Verification items for this drawing (mm, ordinates from the low corner). A direction names the side the tool comes from. Give positions to 0.01 mm unless a question says otherwise; leave off trailing zeros. Loops run counter-clockwise (first coordinate to the right, second up) from the corner with the lowest first, then second, coordinate; pieces in that order, holes last. Notation, with made-up numbers: (69, -3.75) -> (124, -3.75) arc R19 ccw to (124, 4.25) -> close; hole circle Ø7 at (-36.75, -29.5). An arc over 180 degrees is marked (long way). Answer as a JSON object with one key per item and string values.
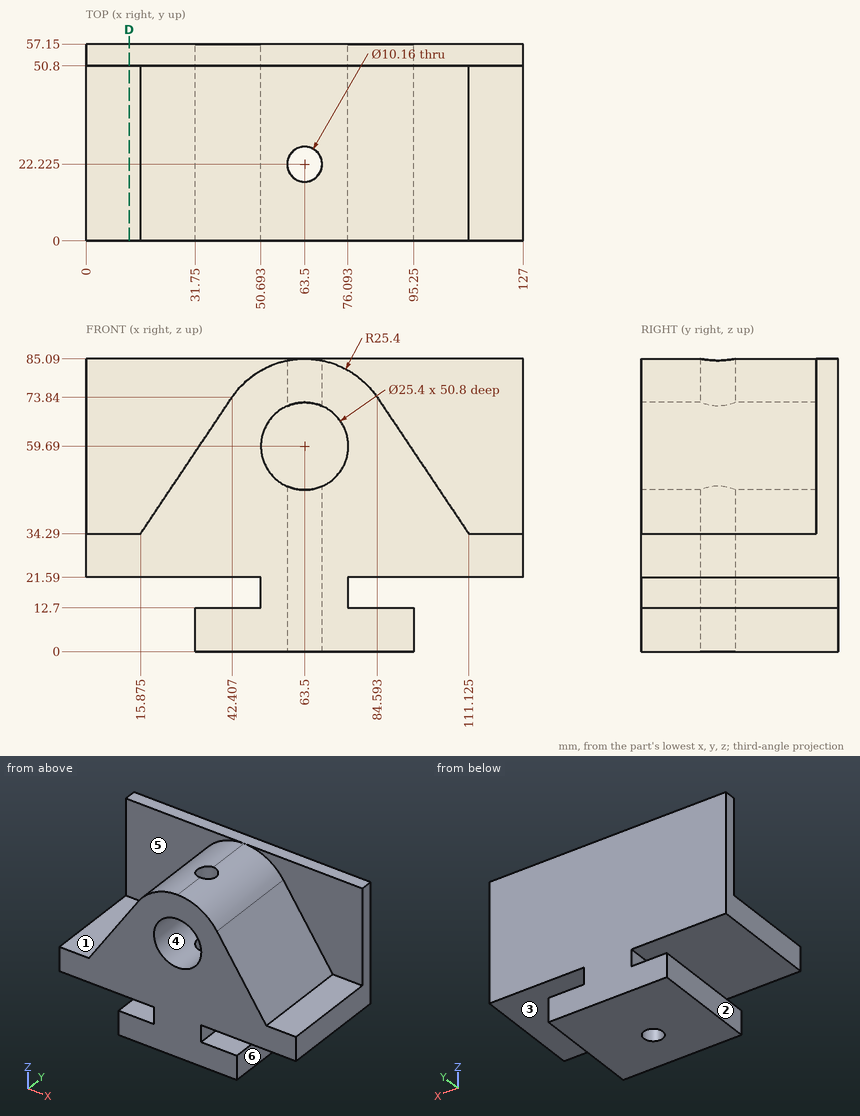
1) Depth check by flat-ended pin: P1, Ø2.5, axis at y = 32, z = 19, coming from the -X side; P2, Ø5.5, axis at x = 84, y = 36, coming from the +Z side; P3, Ø5, axis at x = 10, y = 35, coming from the +Z side. Enter the tip coordinate at first touch or a pass-through.
Geometry check:
{"P1": "stops at x = 50.69", "P2": "stops at z = 77.86", "P3": "stops at z = 34.29"}
2) Section check D-D on x = 12.5. Record the cut outline in (y, z), plus the area to 3 significant figures.
Geometry check:
{"outline": "(0, 21.59) -> (57.15, 21.59) -> (57.15, 85.09) -> (50.8, 85.09) -> (50.8, 34.29) -> (0, 34.29) -> close", "area": "1,050 mm2"}
3) Draft check along X on the marked faces 4, 5 and 6. Enter one of: pulls with the +X half, pulls with the -X half, needs draft (parallel to the pull), parting line crosses it, or undercut.
Geometry check:
{"face 4": "undercut", "face 5": "needs draft", "face 6": "pulls with the +X half"}
4) Tool access check on the marked faces 1, 2 and 3. Record the directions out of +Z, -Z, +X, -X, +Y, -Y that give a thin tool (end or side, any length) a straight path to the whole face; none if there is none.
Geometry check:
{"face 1": "+Z, -X, -Y", "face 2": "-Z, -X, +Y, -Y", "face 3": "+X, +Y, -Y"}
5) Material ranges on line 1 along Y through (x, z) = (63, 76); line 2 along X through (y, z) = (14, 21); line 3 along Z through (x, y) = (36.5, 9.5) (1 decimal), recorded low to high. Write a range as from..to.
Geometry check:
{"line 1": "y = 0..17.17, 27.28..57.15", "line 2": "x = 50.69..76.09", "line 3": "z = 0..12.7, 21.6..65"}
